from build123d import *

# Parameters (mm, degrees)
F1_DEPTH = 3.81
F2_R     = 2.032
F4_DEPTH = 7.621
F5_R     = 0.762
F7_DEPTH = 7.62


# Not quite as in the source:
# - a feature names something its author has since deleted; it is built from what else it names


with BuildPart() as f1:
    # F0 (on Right) → F1 (new body, symmetric)
    with BuildSketch(Plane.YZ):
        with BuildLine():
            Line((0, 43.18), (0, 0))
            Line((0, 0), (0, -5.08))
            Line((0, -5.08), (37.8004340866, -5.08))
            ThreePointArc((37.8004340866, -5.08), (40.7325377806, -4.3625187907), (43.0020495678, -2.3722103708))
            Line((43.0020495678, -2.3722103708), (58.0123892895, 19.0647763833))
            Line((58.0123892895, 19.0647763833), (49.6898045196, 24.8923129766))
            Line((49.6898045196, 24.8923129766), (39.4916154812, 10.3277896292))
            ThreePointArc((39.4916154812, 10.3277896292), (37.222103694, 8.3374812093), (34.29, 7.62))
            Line((34.29, 7.62), (16.51, 7.62))
            ThreePointArc((16.51, 7.62), (12.0198719395, 9.4798719395), (10.16, 13.97))
            Line((10.16, 13.97), (10.16, 43.18))
            Line((10.16, 43.18), (0, 43.18))
        make_face()
    extrude(amount=F1_DEPTH, both=True)

    # F2
    f2_edges = [f1.edges().sort_by_distance(p)[0] for p in [
        (0, 10.16, 43.18),
        (0, 0, 43.18),
        (0, 49.689805, 24.892313),
        (0, 58.012389, 19.064776),
        (0, 0, -5.08),
    ]]
    fillet(f2_edges, radius=F2_R)

    # F3 (on face) → F4 (cut, through all)
    with BuildSketch(Plane.YZ.offset(3.81)):
        with BuildLine():
            Line((6.35, 33.528), (6.35, 37.338))
            ThreePointArc((6.35, 37.338), (5.08, 38.608), (3.81, 37.338))
            Line((3.81, 37.338), (3.81, 30.988))
            Line((3.81, 30.988), (10.16, 30.988))
            Line((10.16, 30.988), (10.16, 33.528))
            Line((10.16, 33.528), (6.35, 33.528))
        make_face()
        with BuildLine():
            Line((6.35, 0.762), (6.35, 7.112))
            ThreePointArc((6.35, 7.112), (5.08, 8.382), (3.81, 7.112))
            Line((3.81, 7.112), (3.81, 3.302))
            Line((3.81, 3.302), (0, 3.302))
            Line((0, 3.302), (0, 0.762))
            Line((0, 0.762), (6.35, 0.762))
        make_face()
    extrude(amount=-F4_DEPTH, mode=Mode.SUBTRACT)

    # F5
    f5_edges = [f1.edges().sort_by_distance(p)[0] for p in [
        (0, 6.35, 33.528),
        (0, 10.16, 33.528),
        (0, 3.81, 30.988),
        (0, 10.16, 30.988),
        (0, 0, 3.302),
        (0, 6.35, 0.762),
        (0, 0, 0.762),
        (0, 3.81, 3.302),
    ]]
    fillet(f5_edges, radius=F5_R)

    # F6 (on face) → F7 (join, through all)
    with BuildSketch(Plane.YZ.offset(3.81)):
        with BuildLine():
            Line((6.35, 35.4090145557), (6.35, 36.6031861632))
            ThreePointArc((6.35, 36.6031861632), (6.1816473942, 36.0061003594), (6.35, 35.4090145557))
        make_face()
        with BuildLine():
            Line((3.81, 36.6031861632), (3.81, 35.4090145557))
            ThreePointArc((3.81, 35.4090145557), (3.9783526058, 36.0061003594), (3.81, 36.6031861632))
        make_face()
        with BuildLine():
            Line((3.81, 6.2505925306), (3.81, 5.0564209231))
            ThreePointArc((3.81, 5.0564209231), (3.9783526058, 5.6535067269), (3.81, 6.2505925306))
        make_face()
        with BuildLine():
            ThreePointArc((6.35, 6.2505925306), (6.1816473942, 5.6535067269), (6.35, 5.0564209231))
            Line((6.35, 5.0564209231), (6.35, 6.2505925306))
        make_face()
    extrude(amount=-F7_DEPTH)


solid = f1.part
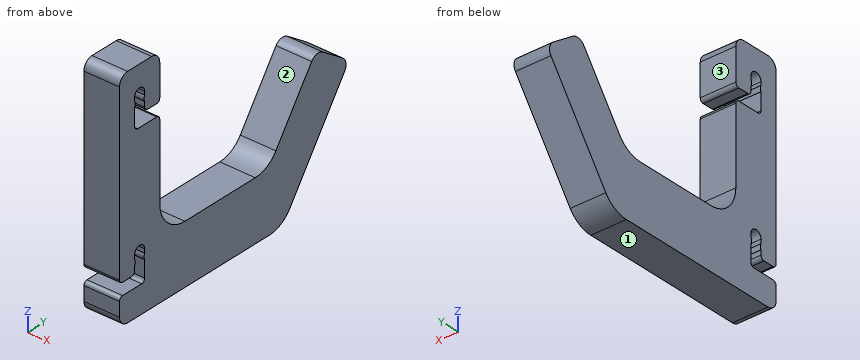
Input: part model. Units: mm. Frame: model coordinates. Face numbers are marked on the shaded views. A direction names the side the tool comes from. Round coordinates to 2 decimals unless told otherwise and drop trailing zeros. Write each loop counter-clockwise with the first axis right and the second up, starting at its lowest first coordinate (ties: lowest second). Pieces come first, ordered by that corner, then holes.
1) Cut plane B-B (y = 25.5). Return the cut outline in (x, z), then the cut area to 3 significant figures.
2) Reachability of the marked faces 1, 2 and 3 from +Z, -Z, +X, -X, +Y, -Y: full face, straight path, thin tool, end or side. Return the list, or none.
3) Contact query for flat-ended pins moving along their axis: P1, Ø2.5, axis at x = 0.5, y = 21.5, coming from the +Z side; P2, Ø1, axis at x = -2, z = 30.5, coming from the +Y side; P3, Ø1.1, axis at x = 0, z = 4.5, coming from the +Y side. Output: stop coordinate, or through.
4) Cut plane C-C (z = 29.5). Return the cut outline in (x, y).
5) Cut plane A-A (z = 19). Return the cut outline in (x, y).
6) Ray query, L1, parallel to Y at x = -2.75, z = 35; L2, parallel to Z at x = -1.5, y = 7; L3, parallel to Z at x = -2, y = 17. Return the intervals inside material, ascending.
Geometry says:
1. outline: (-3.81, -5.08) - (3.81, -5.08) - (3.81, 7.62) - (-3.81, 7.62) - close
1. area: 96.8 mm2
2. face 1: -Z, +X, -X, +Y, -Y
2. face 2: +Z, +X, -X
2. face 3: +Z, +X, -X, +Y
3. P1: stops at z = 7.62
3. P2: stops at y = 10.16
3. P3: stops at y = 48.2
4. outline: (-3.81, 0) - (3.81, 0) - (3.81, 10.16) - (-3.81, 10.16) - close
5. outline: (-3.81, 0) - (3.81, 0) - (3.81, 10.16) - (-3.81, 10.16) - close; (-3.81, 45.56) - (3.81, 45.56) - (3.81, 57.17) - (-3.81, 57.17) - close
6. L1: y = 0 to 3.81, 6.35 to 10.16
6. L2: z = -5.08 to 30.99, 33.54 to 43.18
6. L3: z = -5.08 to 7.62
